Design review of the part built by this model. Coordinates are the model's own, in mm. Coordinates: 2 decimals unless noted, no trailing zeros. Write each loop counter-clockwise with the first axis right and the second up, starting at its lowest first coordinate (ties: lowest second). Pieces come first, ordered by that corner, then holes.
```python
from build123d import *

# Parameters (mm, degrees)
SKETCH1_R                          = 107.5
SKETCH1_R_2                        = 67.5
BOSS_EXTRUDE1_DEPTH                = 3
RIB_SLOT_DEPTH                     = 3
RIB_SLOT_PATTERN_COUNT             = 4
FRONT_BACK_RIB_TAB_CLEARANCE_REACH = 154.041
SKETCH3_W                          = 3.2
SKETCH3_H                          = 5
ELASTIC_ANCHORS_REACH              = 154.041


# Read off the part's stored shape, not the designer's step: rib slot
with BuildPart() as part:
    # Sketch1 → Boss-Extrude1 (new body)
    with BuildSketch(Plane.XY):
        Circle(SKETCH1_R)
        Circle(SKETCH1_R_2, mode=Mode.SUBTRACT)
    extrude(amount=BOSS_EXTRUDE1_DEPTH)

    # rib slot outline → rib slot (cut)
    with BuildSketch(Plane.XY):
        with BuildLine():
            ThreePointArc((-6.135889894, -107.324744841), (-2.287357957, -107.475662331), (1.564110106, -107.488620605))
            Line((1.564110106, -107.488620605), (1.564110106, -93.391745722))
            ThreePointArc((1.564110106, -93.391745722), (2.394190801, -92.114238959), (1, -91.5))
            Line((1, -91.5), (-1, -91.5))
            ThreePointArc((-1, -91.5), (-2.383159214, -92.079561495), (-1.635889894, -93.379795897))
            Line((-1.635889894, -93.379795897), (-1.635889894, -104.5))
            ThreePointArc((-1.635889894, -104.5), (-1.035889894, -105.5), (-1.635889894, -106.5))
            Line((-1.635889894, -106.5), (-4.635889894, -106.5))
            Line((-4.635889894, -106.5), (-4.635889894, -100.5))
            ThreePointArc((-4.635889894, -100.5), (-5.385889894, -99.75), (-6.135889894, -100.5))
            Line((-6.135889894, -100.5), (-6.135889894, -107.324744841))
        make_face()
    rib_slot = extrude(amount=RIB_SLOT_DEPTH, mode=Mode.SUBTRACT)

    # rib slot pattern: rib slot ×4 about axis
    rib_slot_pattern_axis = Axis((0, 0, 0), (0, 0, 1))
    for i in range(1, RIB_SLOT_PATTERN_COUNT):
        add(rib_slot.rotate(rib_slot_pattern_axis, i * 360 / RIB_SLOT_PATTERN_COUNT), mode=Mode.SUBTRACT)

    # Sketch3 → front back rib tab clearance (cut, up to next)
    with BuildSketch(Plane.XY.offset(3), mode=Mode.PRIVATE) as front_back_rib_tab_clearance_sk1:
        with Locations((0, -79)):
            Rectangle(SKETCH3_W, SKETCH3_H)
    front_back_rib_tab_clearance_tool1 = extrude(front_back_rib_tab_clearance_sk1.sketch, amount=-FRONT_BACK_RIB_TAB_CLEARANCE_REACH, mode=Mode.PRIVATE) & part.part
    # Sketch3 → front back rib tab clearance (cut, up to next)
    with BuildSketch(Plane.XY.offset(3), mode=Mode.PRIVATE) as front_back_rib_tab_clearance_sk2:
        with Locations((0, 79)):
            Rectangle(SKETCH3_W, SKETCH3_H)
    front_back_rib_tab_clearance_tool2 = extrude(front_back_rib_tab_clearance_sk2.sketch, amount=-FRONT_BACK_RIB_TAB_CLEARANCE_REACH, mode=Mode.PRIVATE) & part.part
    add(front_back_rib_tab_clearance_tool1.solids().sort_by_distance((0, -79, 3))[0], mode=Mode.SUBTRACT)
    add(front_back_rib_tab_clearance_tool2.solids().sort_by_distance((0, 79, 3))[0], mode=Mode.SUBTRACT)

    # Sketch4 → elastic anchors (cut, up to next)
    with BuildSketch(Plane.XY.offset(3), mode=Mode.PRIVATE) as elastic_anchors_sk1:
        with BuildLine():
            ThreePointArc((-23.570598706, -69.144140951), (-25.601397855, -67.238099637), (-25.446658029, -70.01896178))
            ThreePointArc((-25.446658029, -70.01896178), (-29.075438543, -72.099195538), (-30.948824345, -68.359430018))
            ThreePointArc((-30.948824345, -68.359430018), (-29.143124399, -64.96363906), (-26.471207488, -62.197268051))
            ThreePointArc((-26.471207488, -62.197268051), (-21.930237539, -59.850307494), (-16.846702438, -59.315234774))
            Line((-16.846702438, -59.315234774), (-37.629626544, -51.750869019))
            ThreePointArc((-37.629626544, -51.750869019), (-34.079350843, -55.428391879), (-32.109363213, -60.145147191))
            ThreePointArc((-32.109363213, -60.145147191), (-31.84074512, -63.981785414), (-32.640271063, -67.74379376))
            ThreePointArc((-32.640271063, -67.74379376), (-28.95818762, -73.967017614), (-23.570598706, -69.144140951))
        make_face()
    elastic_anchors_tool1 = extrude(elastic_anchors_sk1.sketch, amount=-ELASTIC_ANCHORS_REACH, mode=Mode.PRIVATE) & part.part
    # Sketch4 → elastic anchors (cut, up to next)
    with BuildSketch(Plane.XY.offset(3), mode=Mode.PRIVATE) as elastic_anchors_sk2:
        with BuildLine():
            ThreePointArc((23.570598706, -69.144140951), (25.601397855, -67.238099637), (25.446658029, -70.01896178))
            ThreePointArc((25.446658029, -70.01896178), (29.075438543, -72.099195538), (30.948824345, -68.359430018))
            ThreePointArc((30.948824345, -68.359430018), (29.143124399, -64.96363906), (26.471207488, -62.197268051))
            ThreePointArc((26.471207488, -62.197268051), (21.930237539, -59.850307494), (16.846702438, -59.315234774))
            Line((16.846702438, -59.315234774), (37.629626544, -51.750869019))
            ThreePointArc((37.629626544, -51.750869019), (34.079350843, -55.428391879), (32.109363213, -60.145147191))
            ThreePointArc((32.109363213, -60.145147191), (31.84074512, -63.981785414), (32.640271063, -67.74379376))
            ThreePointArc((32.640271063, -67.74379376), (28.95818762, -73.967017614), (23.570598706, -69.144140951))
        make_face()
    elastic_anchors_tool2 = extrude(elastic_anchors_sk2.sketch, amount=-ELASTIC_ANCHORS_REACH, mode=Mode.PRIVATE) & part.part
    # Sketch4 → elastic anchors (cut, up to next)
    with BuildSketch(Plane.XY.offset(3), mode=Mode.PRIVATE) as elastic_anchors_sk3:
        with BuildLine():
            ThreePointArc((-69.144140951, 23.570598706), (-67.238099637, 25.601397855), (-70.01896178, 25.446658029))
            ThreePointArc((-70.01896178, 25.446658029), (-72.099195538, 29.075438543), (-68.359430018, 30.948824345))
            ThreePointArc((-68.359430018, 30.948824345), (-64.96363906, 29.143124399), (-62.197268051, 26.471207488))
            ThreePointArc((-62.197268051, 26.471207488), (-59.850307494, 21.930237539), (-59.315234774, 16.846702438))
            Line((-59.315234774, 16.846702438), (-51.750869019, 37.629626544))
            ThreePointArc((-51.750869019, 37.629626544), (-55.428391879, 34.079350843), (-60.145147191, 32.109363213))
            ThreePointArc((-60.145147191, 32.109363213), (-63.981785414, 31.84074512), (-67.74379376, 32.640271063))
            ThreePointArc((-67.74379376, 32.640271063), (-73.967017614, 28.95818762), (-69.144140951, 23.570598706))
        make_face()
    elastic_anchors_tool3 = extrude(elastic_anchors_sk3.sketch, amount=-ELASTIC_ANCHORS_REACH, mode=Mode.PRIVATE) & part.part
    # Sketch4 → elastic anchors (cut, up to next)
    with BuildSketch(Plane.XY.offset(3), mode=Mode.PRIVATE) as elastic_anchors_sk4:
        with BuildLine():
            ThreePointArc((-69.144140951, -23.570598706), (-67.238099637, -25.601397855), (-70.01896178, -25.446658029))
            ThreePointArc((-70.01896178, -25.446658029), (-72.099195538, -29.075438543), (-68.359430018, -30.948824345))
            ThreePointArc((-68.359430018, -30.948824345), (-64.96363906, -29.143124399), (-62.197268051, -26.471207488))
            ThreePointArc((-62.197268051, -26.471207488), (-59.850307494, -21.930237539), (-59.315234774, -16.846702438))
            Line((-59.315234774, -16.846702438), (-51.750869019, -37.629626544))
            ThreePointArc((-51.750869019, -37.629626544), (-55.428391879, -34.079350843), (-60.145147191, -32.109363213))
            ThreePointArc((-60.145147191, -32.109363213), (-63.981785414, -31.84074512), (-67.74379376, -32.640271063))
            ThreePointArc((-67.74379376, -32.640271063), (-73.967017614, -28.95818762), (-69.144140951, -23.570598706))
        make_face()
    elastic_anchors_tool4 = extrude(elastic_anchors_sk4.sketch, amount=-ELASTIC_ANCHORS_REACH, mode=Mode.PRIVATE) & part.part
    # Sketch4 → elastic anchors (cut, up to next)
    with BuildSketch(Plane.XY.offset(3), mode=Mode.PRIVATE) as elastic_anchors_sk5:
        with BuildLine():
            ThreePointArc((23.570598706, 69.144140951), (25.601397855, 67.238099637), (25.446658029, 70.01896178))
            ThreePointArc((25.446658029, 70.01896178), (29.075438543, 72.099195538), (30.948824345, 68.359430018))
            ThreePointArc((30.948824345, 68.359430018), (29.143124399, 64.96363906), (26.471207488, 62.197268051))
            ThreePointArc((26.471207488, 62.197268051), (21.930237539, 59.850307494), (16.846702438, 59.315234774))
            Line((16.846702438, 59.315234774), (37.629626544, 51.750869019))
            ThreePointArc((37.629626544, 51.750869019), (34.079350843, 55.428391879), (32.109363213, 60.145147191))
            ThreePointArc((32.109363213, 60.145147191), (31.84074512, 63.981785414), (32.640271063, 67.74379376))
            ThreePointArc((32.640271063, 67.74379376), (28.95818762, 73.967017614), (23.570598706, 69.144140951))
        make_face()
    elastic_anchors_tool5 = extrude(elastic_anchors_sk5.sketch, amount=-ELASTIC_ANCHORS_REACH, mode=Mode.PRIVATE) & part.part
    # Sketch4 → elastic anchors (cut, up to next)
    with BuildSketch(Plane.XY.offset(3), mode=Mode.PRIVATE) as elastic_anchors_sk6:
        with BuildLine():
            ThreePointArc((-23.570598706, 69.144140951), (-25.601397855, 67.238099637), (-25.446658029, 70.01896178))
            ThreePointArc((-25.446658029, 70.01896178), (-29.075438543, 72.099195538), (-30.948824345, 68.359430018))
            ThreePointArc((-30.948824345, 68.359430018), (-29.143124399, 64.96363906), (-26.471207488, 62.197268051))
            ThreePointArc((-26.471207488, 62.197268051), (-21.930237539, 59.850307494), (-16.846702438, 59.315234774))
            Line((-16.846702438, 59.315234774), (-37.629626544, 51.750869019))
            ThreePointArc((-37.629626544, 51.750869019), (-34.079350843, 55.428391879), (-32.109363213, 60.145147191))
            ThreePointArc((-32.109363213, 60.145147191), (-31.84074512, 63.981785414), (-32.640271063, 67.74379376))
            ThreePointArc((-32.640271063, 67.74379376), (-28.95818762, 73.967017614), (-23.570598706, 69.144140951))
        make_face()
    elastic_anchors_tool6 = extrude(elastic_anchors_sk6.sketch, amount=-ELASTIC_ANCHORS_REACH, mode=Mode.PRIVATE) & part.part
    # Sketch4 → elastic anchors (cut, up to next)
    with BuildSketch(Plane.XY.offset(3), mode=Mode.PRIVATE) as elastic_anchors_sk7:
        with BuildLine():
            ThreePointArc((69.144140951, -23.570598706), (67.238099637, -25.601397855), (70.01896178, -25.446658029))
            ThreePointArc((70.01896178, -25.446658029), (72.099195538, -29.075438543), (68.359430018, -30.948824345))
            ThreePointArc((68.359430018, -30.948824345), (64.96363906, -29.143124399), (62.197268051, -26.471207488))
            ThreePointArc((62.197268051, -26.471207488), (59.850307494, -21.930237539), (59.315234774, -16.846702438))
            Line((59.315234774, -16.846702438), (51.750869019, -37.629626544))
            ThreePointArc((51.750869019, -37.629626544), (55.428391879, -34.079350843), (60.145147191, -32.109363213))
            ThreePointArc((60.145147191, -32.109363213), (63.981785414, -31.84074512), (67.74379376, -32.640271063))
            ThreePointArc((67.74379376, -32.640271063), (73.967017614, -28.95818762), (69.144140951, -23.570598706))
        make_face()
    elastic_anchors_tool7 = extrude(elastic_anchors_sk7.sketch, amount=-ELASTIC_ANCHORS_REACH, mode=Mode.PRIVATE) & part.part
    # Sketch4 → elastic anchors (cut, up to next)
    with BuildSketch(Plane.XY.offset(3), mode=Mode.PRIVATE) as elastic_anchors_sk8:
        with BuildLine():
            ThreePointArc((69.144140951, 23.570598706), (67.238099637, 25.601397855), (70.01896178, 25.446658029))
            ThreePointArc((70.01896178, 25.446658029), (72.099195538, 29.075438543), (68.359430018, 30.948824345))
            ThreePointArc((68.359430018, 30.948824345), (64.96363906, 29.143124399), (62.197268051, 26.471207488))
            ThreePointArc((62.197268051, 26.471207488), (59.850307494, 21.930237539), (59.315234774, 16.846702438))
            Line((59.315234774, 16.846702438), (51.750869019, 37.629626544))
            ThreePointArc((51.750869019, 37.629626544), (55.428391879, 34.079350843), (60.145147191, 32.109363213))
            ThreePointArc((60.145147191, 32.109363213), (63.981785414, 31.84074512), (67.74379376, 32.640271063))
            ThreePointArc((67.74379376, 32.640271063), (73.967017614, 28.95818762), (69.144140951, 23.570598706))
        make_face()
    elastic_anchors_tool8 = extrude(elastic_anchors_sk8.sketch, amount=-ELASTIC_ANCHORS_REACH, mode=Mode.PRIVATE) & part.part
    add(elastic_anchors_tool1.solids().sort_by_distance((-28.423672, -62.033014, 3))[0], mode=Mode.SUBTRACT)
    add(elastic_anchors_tool2.solids().sort_by_distance((28.423672, -62.033014, 3))[0], mode=Mode.SUBTRACT)
    add(elastic_anchors_tool3.solids().sort_by_distance((-62.033014, 28.423672, 3))[0], mode=Mode.SUBTRACT)
    add(elastic_anchors_tool4.solids().sort_by_distance((-62.033014, -28.423672, 3))[0], mode=Mode.SUBTRACT)
    add(elastic_anchors_tool5.solids().sort_by_distance((28.423672, 62.033014, 3))[0], mode=Mode.SUBTRACT)
    add(elastic_anchors_tool6.solids().sort_by_distance((-28.423672, 62.033014, 3))[0], mode=Mode.SUBTRACT)
    add(elastic_anchors_tool7.solids().sort_by_distance((62.033014, -28.423672, 3))[0], mode=Mode.SUBTRACT)
    add(elastic_anchors_tool8.solids().sort_by_distance((62.033014, 28.423672, 3))[0], mode=Mode.SUBTRACT)


solid = part.part
```
(1) Consider section C-C (z = 0.5). State how many separate pieces and enclosed holes the cut face has, plus the area to 3 significant figures.
(2) Mouldability with a two-part tool opening along X and no side actions: class faces 1 (the cylindrical face through (-73.95, -29.07, 1.52)), 2 (the cylindrical face through (-47.92, -47.54, 1.48)), 3 (the flat face through (-2, -70, 3)), 4 (the cylindrical face through (78.39, 73.56, 1.48)) as +X half, -X half, draft (parallel to the pull), parting line (faces both ways), or undercut.
(3) Insertion check: pin 1 Ø10 at (x, y) = (38.5, 46) entering from -Z; pin 2 Ø1.5 at (y, z) = (-30, 1) entering from +X; pin 3 Ø0.6 at (x, z) = (0, 2) entering from -Y; pin 4 Ø0.9 at (x, z) = (-99.5, 2) entering from +Y. Each pin has a flat end and moves straight along its axis. Give the tip position at first contact, or say it passes through.
(4) Consider section A-A (y = -79). Give the boundary of the cut face in (x, z), plus the area to 3 significant figures.
(5) Consider section B-B (x = -45.5). Give the boundary of the cut face in (y, z).
(6) Wall thickness on line 1 (Y direction, x = -69.5, z = 2.7); line 2 (Y direction, x = -25, z = 2.45); line 3 (X direction, y = -70, z = 2.15): over which ranges is each line inside the solid? List them lowest first.
Results:
1. separate pieces: 1
1. enclosed holes: 3
1. area: 21,300 mm2
2. face 1: undercut
2. face 2: undercut
2. face 3: draft
2. face 4: +X half
3. pin 1: passes through
3. pin 2: stops at x = 103.44
3. pin 3: stops at y = -91.5
3. pin 4: stops at y = 41.78
4. outline: (-72.91, 0) - (-1.6, 0) - (-1.6, 3) - (-72.91, 3) - close; (1.6, 0) - (72.91, 0) - (72.91, 3) - (1.6, 3) - close
4. area: 428 mm2
5. outline: (-97.4, 0) - (-49.86, 0) - (-49.86, 3) - (-97.4, 3) - close; (49.86, 0) - (97.4, 0) - (97.4, 3) - (49.86, 3) - close
6. line 1: y = -82.01 to -32.92, -31.12 to -26.17, -23.57 to 23.57, 26.17 to 31.12, 32.92 to 82.01
6. line 2: y = -104.55 to -72.71, -67.1 to -62.7, 62.7 to 67.1, 72.71 to 104.55
6. line 3: x = -81.59 to -32.88, -31.05 to -25.5, -23.61 to 23.61, 25.5 to 31.05, 32.88 to 81.59
